The drawing under review shows one solid part. Ordinate dimensions are in mm from its lowest x, y, z. A direction names the side the tool comes from. Coordinates: 2 decimals unless noted, no trailing zeros. Loops run counter-clockwise (first coordinate to the right, second up) from the corner with the lowest first, then second, coordinate; pieces in that order, holes last. Notation, with made-up numbers: M 10.5,79.25 L 46.5,79.25 A21 ccw 46.5,109.25 Z; hole C 29,35 d8. An arc over 180 degrees is marked long. Answer as a JSON object with one key per item and string values. Group by question number.
1. To check wall thickness, follow probe 1 along Y at (x, z) = (7, 5); probe 2 along Y at (x, z) = (30, 7); probe 3 along X at (y, z) = (55, 21.5). State the ranges of each line that lie inside material, in increasing order.
2. Consider section D-D (x = 7.5). State the section outline as (y, z) points.
3. Consider section A-A (z = 40). State the section outline as (x, y) points, then the cut area to 3 significant figures.
4. Consider section B-B (y = 50). State the section outline as (x, z) points.
5. Consider section C-C (x = 30). State the section outline as (y, z) points, then the cut area to 3 significant figures.
6. Machinability: for the marked faces 1 and 2, which of the approach directions +Z, -Z, +X, -X, +Y, -Y give a long, thin tool a straight path to every point of the face, cutting with its end or side? Answer none if there is none.
7. Insertion check: pin 1 (10 mm diameter, centred on y = 79, z = 35, fed in from -X). The pin has a flat end and moves straight along its axis. Give the tip position at first contact, or say it passes through.
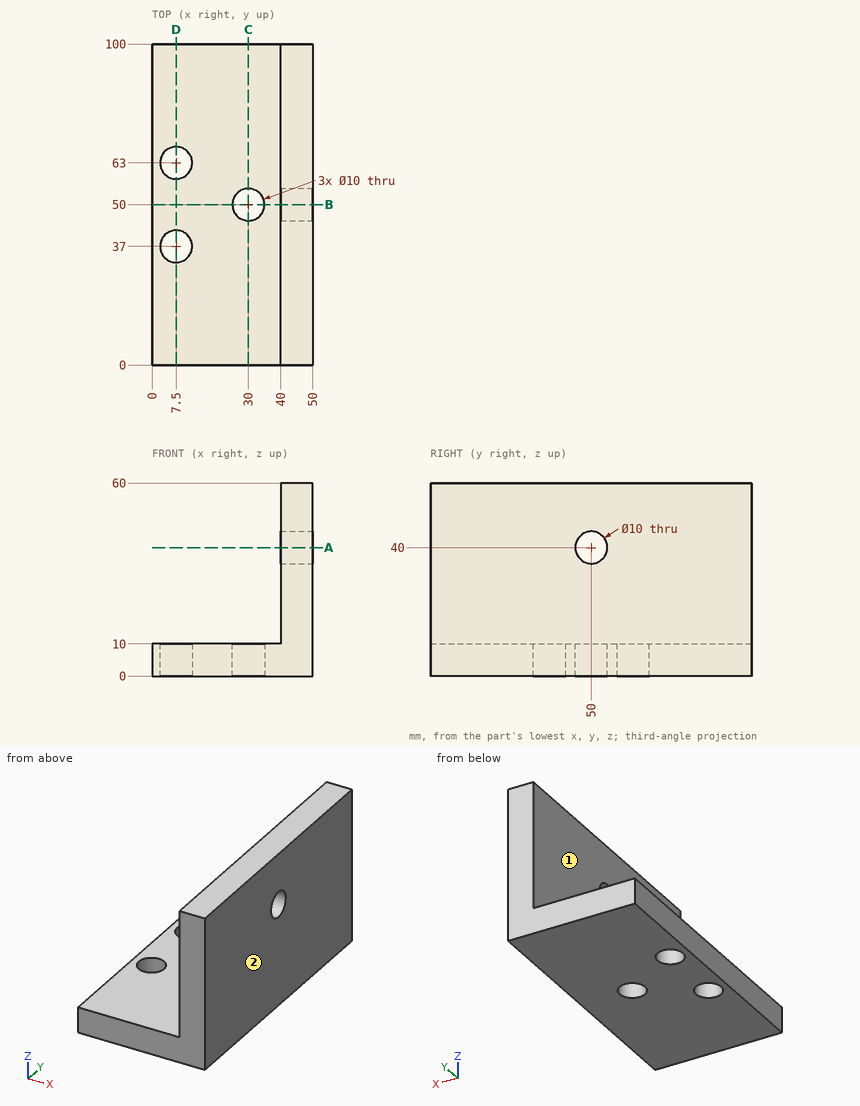
Findings below:
{
 "1": {"probe 1": "y = 0 to 32.03, 41.97 to 58.03, 67.97 to 100", "probe 2": "y = 0 to 45, 55 to 100", "probe 3": "x = 40 to 50"},
 "2": {"outline": "M 0,0 L 32,0 L 32,10 L 0,10 Z; M 42,0 L 58,0 L 58,10 L 42,10 Z; M 68,0 L 100,0 L 100,10 L 68,10 Z"},
 "3": {"outline": "M 40,0 L 50,0 L 50,45 L 40,45 Z; M 40,55 L 50,55 L 50,100 L 40,100 Z", "area": "900 mm^2"},
 "4": {"outline": "M 0,0 L 25,0 L 25,10 L 0,10 Z; M 35,0 L 50,0 L 50,35 L 40,35 L 40,10 L 35,10 Z; M 40,45 L 50,45 L 50,60 L 40,60 Z"},
 "5": {"outline": "M 0,0 L 45,0 L 45,10 L 0,10 Z; M 55,0 L 100,0 L 100,10 L 55,10 Z", "area": "900 mm^2"},
 "6": {"face 1": "+Z, -X, +Y, -Y", "face 2": "+Z, -Z, +X, +Y, -Y"},
 "7": {"pin 1": "stops at x = 40"}
}
